Here's how the part is built. I have some questions about the finished solid (model axes, mm). Coordinates: 2 decimals unless noted, no trailing zeros. Loops run counter-clockwise (first coordinate to the right, second up) from the corner with the lowest first, then second, coordinate; pieces in that order, holes last. Notation, with made-up numbers: (67.25, 73.5) -> (120.25, 73.5) arc R28 cw to (120.25, 93.5) -> close; hole circle Ø3 at (59.25, 3). An arc over 180 degrees is marked (long way). Answer as a JSON object with one key per item and string values. Group by question number.
1) I need wall thicknesses on probe 1 along X at (y, z) = (90.5, 0.9); probe 2 along X at (y, z) = (58, 0.5); probe 3 along Y at (x, z) = (27.5, 2.1). Which ranges of each line are inside material? Lowest first, please. Write a range as [from, to].
2) I want a section at A-A (y = -76). Write out the boundary of the cut face in (x, z).
3) I'm going to push flat-ended pins straight in: pin 1 (1.6 mm diameter, centred on x = 3, z = 1.5, fed in from -Y); pin 2 (1.6 mm diameter, centred on x = -102.5, z = 2, fed in from -Y); pin 3 (1.3 mm diameter, centred on y = -93.5, z = 1, fed in from +X). Where does each tip first touch, or does it pass through?
```python
from build123d import *

# Parameters (mm, degrees)
SKETCH2_W           = 200
SKETCH2_H           = 200
BOSS_EXTRUDE1_DEPTH = 3.18
CUT_EXTRUDE1_DEPTH  = 142.457104452
SKETCH4_W           = 3.18
SKETCH4_H           = 10
BOSS_EXTRUDE2_DEPTH = 3.18
SKETCH6_R           = 1.47
CUT_EXTRUDE2_DEPTH  = 144.722735849
SKETCH7_R           = 1.6
CUT_EXTRUDE3_DEPTH  = 144.722735849


with BuildPart() as part:
    # Sketch2 → Boss-Extrude1 (new body)
    with BuildSketch(Plane.XY):
        Rectangle(SKETCH2_W, SKETCH2_H)
    extrude(amount=BOSS_EXTRUDE1_DEPTH)

    # Sketch3 → Cut-Extrude1 (cut, through all)
    with BuildSketch(Plane.XY.offset(3.18)):
        Polygon((-5, 100), (5, 100), (5, 96.82), (1.47, 96.82), (1.47, 94.74), (3.25, 94.74), (3.25, 92.14), (1.47, 92.14), (1.47, 90.07), (-1.47, 90.07), (-1.47, 92.14), (-3.25, 92.14), (-3.25, 94.74), (-1.47, 94.74), (-1.47, 96.82), (-5, 96.82), align=None)
        Polygon((1.47, -96.82), (5, -96.82), (5, -100), (-5, -100), (-5, -96.82), (-1.47, -96.82), (-1.47, -94.74), (-3.25, -94.74), (-3.25, -92.14), (-1.47, -92.14), (-1.47, -90.07), (1.47, -90.07), (1.47, -92.14), (3.25, -92.14), (3.25, -94.74), (1.47, -94.74), align=None)
    extrude(amount=-CUT_EXTRUDE1_DEPTH, mode=Mode.SUBTRACT)

    # Sketch4 → Boss-Extrude2 (add)
    with BuildSketch(Plane.ZY.offset(100)):
        with Locations((1.59, 0)):
            Rectangle(SKETCH4_W, SKETCH4_H)
    boss_extrude2 = extrude(amount=BOSS_EXTRUDE2_DEPTH)

    # Sketch6 → Cut-Extrude2 (cut, through all)
    with BuildSketch(Plane.XY.offset(3.18)):
        with Locations((-101.43, 0)):
            Circle(SKETCH6_R)
    cut_extrude2 = extrude(amount=-CUT_EXTRUDE2_DEPTH, mode=Mode.SUBTRACT)

    # Mirror1: Boss-Extrude2 across plane
    add(boss_extrude2.mirror(Plane(origin=(0, 0, 0), x_dir=(0, 0, 1), z_dir=(1, 0, 0))))

    # Mirror2: Cut-Extrude2 across plane
    add(cut_extrude2.mirror(Plane(origin=(0, 0, 0), x_dir=(0, 0, 1), z_dir=(1, 0, 0))), mode=Mode.SUBTRACT)

    # Sketch7 → Cut-Extrude3 (cut, through all)
    with BuildSketch(Plane.XY.offset(3.18)):
        with Locations((26.179371117, -54.817968537)):
            Circle(SKETCH7_R)
        with Locations((26.179371117, -26.917968537)):
            Circle(SKETCH7_R)
        with Locations((-24.620628883, -11.617968537)):
            Circle(SKETCH7_R)
        with Locations((-26.220628883, -59.917968537)):
            Circle(SKETCH7_R)
    extrude(amount=-CUT_EXTRUDE3_DEPTH, mode=Mode.SUBTRACT)


solid = part.part
```
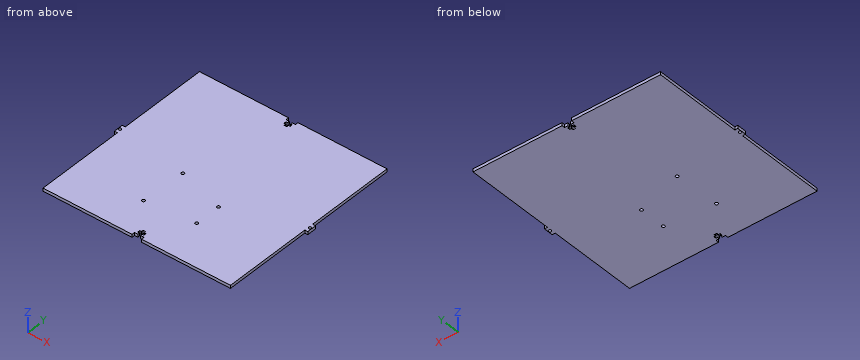
Determined:
{
 "1": {"probe 1": "[-100, -1.47], [1.47, 100]", "probe 2": "[-100, 100]", "probe 3": "[-100, -55.72], [-53.91, -27.82], [-26.01, 100]"},
 "2": {"outline": "(-100, 0) -> (100, 0) -> (100, 3.18) -> (-100, 3.18) -> close"},
 "3": {"pin 1": "y = -96.82", "pin 2": "y = -5", "pin 3": "x = 100"}
}
